from build123d import *

# Parameters (mm, degrees)
SALIENTE_EXTRUIR1_DEPTH = 15
CROQUIS2_R              = 16.164040976
SALIENTE_EXTRUIR2_DEPTH = 25
CROQUIS4_R              = 12.514075771
CORTAR_EXTRUIR1_DEPTH   = 61


with BuildPart() as part:
    # Croquis1 → Saliente-Extruir1 (new body)
    with BuildSketch(Plane(origin=(0, 0, 0), x_dir=(1, 0, 0), z_dir=(0, 1, 0))):
        Polygon((22.5, 0), (11.25, 19.485571585), (-11.25, 19.485571585), (-22.5, 0), (-11.25, -19.485571585), (11.25, -19.485571585), align=None)
    extrude(amount=SALIENTE_EXTRUIR1_DEPTH)

    # Croquis2 → Saliente-Extruir2 (add)
    with BuildSketch(Plane.XZ):
        Circle(CROQUIS2_R)
    extrude(amount=SALIENTE_EXTRUIR2_DEPTH)

    # Croquis4 → Cortar-Extruir1 (cut, through all)
    with BuildSketch(Plane.XZ.offset(45)):
        Circle(CROQUIS4_R)
    extrude(amount=-CORTAR_EXTRUIR1_DEPTH, mode=Mode.SUBTRACT)


solid = part.part
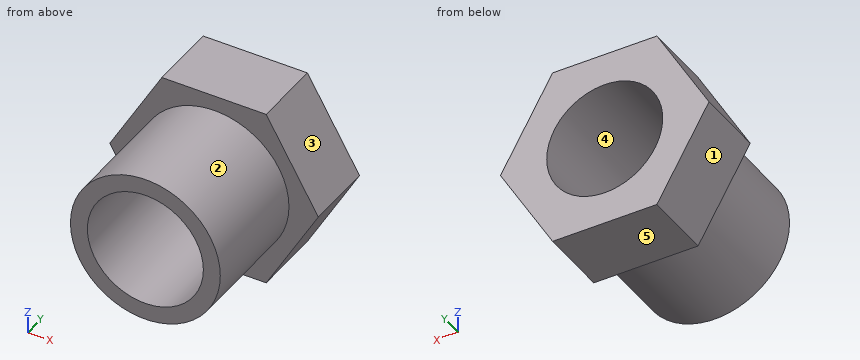
Check sheet for the modelled part. Datum: model origin and axes. Units: mm. Face numbers are marked on the shaded views. A direction names the side the tool comes from. Give positions to 0.01 mm unless a question says otherwise; leave off trailing zeros. Loops run counter-clockwise (first coordinate to the right, second up) from the corner with the lowest first, then second, coordinate; pieces in that order, holes last. Notation, with made-up numbers: M 61.5,50 L 97.5,50 A9 cw 97.5,63 Z; hole C -27.5,74.25 d10. An arc over 180 degrees is marked long. Answer as a JSON object with one key per item and string values. Group by question number.
Q1. Material ranges on line 1 along Z through (x, y) = (0, -2.5); line 2 along Z through (x, y) = (0, 2); line 3 along Z through (x, y) = (-16, 6), recorded low to high. Write a range as [from, to].
Q2. Go/stop test with flat-tipped pins: P1, Ø5, axis at x = -16, y = -6.5, coming from the -Z side; P2, Ø8, axis at y = -5, z = 12, coming from the +X side; P3, Ø8, axis at y = 8.5, z = -4.5, coming from the +X side; P4, Ø3, axis at x = 11.5, z = 12, coming from the -Y side. Record where each tip stops, or that it passes through.
Q3. Access from +Z, -Z, +X, -X, +Y, -Y to the whole of each face (thin tool, end or side, straight path). Record for the marked faces 1 and 2.
Q4. Cross-section at A-A on x = 0. Record the cut outline in (y, z), then the cut area to 3 significant figures.
Q5. Cross-section at B-B on z = -3. Record the cut outline in (x, y).
Q6. Release check for a two-part mould opening along X. For the marked faces 3, 4 and 5 record: released by +X, released by -X, zero draft, split by the parting line, or undercut.
Q7. Cross-section at D-D on z = 15. Record the cut outline in (x, y), then the cut area to 3 significant figures.
Q8. Cross-section at C-C on y = -3.5. Record the cut outline in (x, z).
Evaluation:
{
 "1": {"line 1": "z = [-16.16, -12.51], [12.51, 16.16]", "line 2": "z = [-19.49, -12.51], [12.51, 19.49]", "line 3": "z = [-11.26, 11.26]"},
 "2": {"P1": "stops at z = -8.89", "P2": "stops at x = 14.05", "P3": "stops at x = 22.21", "P4": "stops at y = -25"},
 "3": {"face 1": "-Z, -X, +Y, -Y", "face 2": "-Y"},
 "4": {"outline": "M -25,-16.16 L 0,-16.16 L 0,-19.49 L 15,-19.49 L 15,-12.51 L -25,-12.51 Z; M -25,12.51 L 15,12.51 L 15,19.49 L 0,19.49 L 0,16.16 L -25,16.16 Z", "area": "392 mm2"},
 "5": {"outline": "M -20.77,0 L -15.88,0 L -15.88,-25 L -12.15,-25 L -12.15,15 L -20.77,15 Z; M 12.15,-25 L 15.88,-25 L 15.88,0 L 20.77,0 L 20.77,15 L 12.15,15 Z"},
 "6": {"face 3": "released by +X", "face 4": "undercut", "face 5": "zero draft"},
 "7": {"outline": "M -13.84,0 L -6.02,0 L -6.02,-25 L 6.02,-25 L 6.02,0 L 13.84,0 L 13.84,15 L -13.84,15 Z", "area": "716 mm2"},
 "8": {"outline": "C 0,0 d32.33; hole C 0,0 d25.03"}
}
